```python
from build123d import *

# Parameters (mm, degrees)
SKETCH1_R                                      = 19.05
BOSS_EXTRUDE1_DEPTH                            = 9.525
SKETCH2_W                                      = 1.89865
SKETCH2_H                                      = 43.65625
F_10_CLEARANCE_HOLE1_D                         = 5.1054
F_10_CLEARANCE_HOLE1_DEPTH                     = 11.90625
F_10_CLEARANCE_HOLE2_D                         = 5.1054
F_10_CLEARANCE_HOLE2_DEPTH                     = 11.90625
F_10_24_TAPPED_HOLE2_D                         = 3.7973
F_10_24_TAPPED_HOLE3_D                         = 3.7973
F_10_24_TAPPED_HOLE3_DEPTH                     = 14.986
F_10_24_TAPPED_HOLE3_TIP                       = 1.140824014
CBORE_FOR_8_SOCKET_HEAD_CAP_SCREW1_D           = 4.9149
CBORE_FOR_8_SOCKET_HEAD_CAP_SCREW1_CBORE_D     = 7.9375
CBORE_FOR_8_SOCKET_HEAD_CAP_SCREW1_CBORE_DEPTH = 16.8656
CBORE_FOR_8_SOCKET_HEAD_CAP_SCREW2_D           = 4.9149
CBORE_FOR_8_SOCKET_HEAD_CAP_SCREW2_CBORE_D     = 7.9375
CBORE_FOR_8_SOCKET_HEAD_CAP_SCREW2_CBORE_DEPTH = 5.4356
F_8_32_TAPPED_HOLE1_D                          = 3.4544
F_8_32_TAPPED_HOLE1_DEPTH                      = 12.446
F_8_32_TAPPED_HOLE1_TIP                        = 1.037806461
F_8_32_TAPPED_HOLE2_D                          = 3.4544


with BuildPart() as part:
    # Sketch1 → Boss-Extrude1 (new body)
    with BuildSketch(Plane(origin=(0, 0, 0), x_dir=(1, 0, 0), z_dir=(0, 1, 0))):
        with BuildLine():
            Line((120.206642486, 6.011694636), (120.206642486, 17.917944636))
            Line((120.206642486, 17.917944636), (110.631837795, 17.917944636))
            ThreePointArc((110.631837795, 17.917944636), (97.981642486, 18.711694636), (110.631837795, 19.505444636))
            Line((110.631837795, 19.505444636), (120.206642486, 19.505444636))
            Line((120.206642486, 19.505444636), (120.206642486, 31.411694636))
            Line((120.206642486, 31.411694636), (-438.593357514, 31.411694636))
            Line((-438.593357514, 31.411694636), (-438.593357514, 19.505444636))
            Line((-438.593357514, 19.505444636), (-429.018552824, 19.505444636))
            ThreePointArc((-429.018552824, 19.505444636), (-416.368357514, 18.711694636), (-429.018552824, 17.917944636))
            Line((-429.018552824, 17.917944636), (-438.593357514, 17.917944636))
            Line((-438.593357514, 17.917944636), (-438.593357514, 6.011694636))
            Line((-438.593357514, 6.011694636), (37.656642486, 6.011694636))
            Line((37.656642486, 6.011694636), (37.656642486, -25.738305364))
            Line((37.656642486, -25.738305364), (94.806642486, -25.738305364))
            Line((94.806642486, -25.738305364), (94.806642486, 6.011694636))
            Line((94.806642486, 6.011694636), (120.206642486, 6.011694636))
        make_face()
        with Locations(Location((66.231642486, 2.836694636, 0), (0, 0, 90))):
            Circle(SKETCH1_R, mode=Mode.SUBTRACT)
    extrude(amount=BOSS_EXTRUDE1_DEPTH)

    # Sketch2 → #10-24 Tapped Hole1 (revolve, cut)
    with BuildSketch(Plane(origin=(115.444142486, 4.7625, -17.917944636), x_dir=(0, 1, 0), z_dir=(1, 0, 0))):
        with Locations((0.949325, 21.828125)):
            Rectangle(SKETCH2_W, SKETCH2_H)
    revolve(axis=Axis((115.444142486, 4.7625, -24.267944636), (0, 0, 1)), mode=Mode.SUBTRACT)

    # #10 Clearance Hole1
    with Locations(Plane(origin=(0, 0, -31.411694636), x_dir=(-1, 0, 0), z_dir=(0, 0, -1))):
        with Locations((-115.444142486, 4.7625)):
            Hole(F_10_CLEARANCE_HOLE1_D / 2, depth=F_10_CLEARANCE_HOLE1_DEPTH)

    # #10 Clearance Hole2
    with Locations(Plane(origin=(0, 0, -31.411694636), x_dir=(-1, 0, 0), z_dir=(0, 0, -1))):
        with Locations((433.830857514, 4.7625)):
            Hole(F_10_CLEARANCE_HOLE2_D / 2, depth=F_10_CLEARANCE_HOLE2_DEPTH)

    # #10-24 Tapped Hole2 (through all)
    with Locations(Plane(origin=(0, 0, -17.917944636), x_dir=(-1, 0, 0), z_dir=(0, 0, -1))):
        with Locations((433.830857514, 4.7625)):
            Hole(F_10_24_TAPPED_HOLE2_D / 2)

    # #10-24 Tapped Hole3
    with Locations(Plane(origin=(0, 0, 0), x_dir=(-1, 0, 0), z_dir=(0, -1, 0))):
        with Locations((-89.802842486, 26.407894636), (-42.660442486, 26.407894636), (-42.660442486, -20.734505364), (-89.802842486, -20.734505364)):
            Hole(F_10_24_TAPPED_HOLE3_D / 2, depth=F_10_24_TAPPED_HOLE3_DEPTH)
            with Locations((0, 0, -(F_10_24_TAPPED_HOLE3_DEPTH + F_10_24_TAPPED_HOLE3_TIP / 2))):  # 118° drill point
                Cone(0, F_10_24_TAPPED_HOLE3_D / 2, F_10_24_TAPPED_HOLE3_TIP, mode=Mode.SUBTRACT)

    # CBORE for #8 Socket Head Cap Screw1 (through all)
    with Locations(Plane(origin=(0, 0, -31.411694636), x_dir=(-1, 0, 0), z_dir=(0, 0, -1))):
        with Locations((-31.306642486, 4.7625), (-18.606642486, 4.7625), (406.843357514, 4.7625), (394.143357514, 4.7625)):
            CounterBoreHole(CBORE_FOR_8_SOCKET_HEAD_CAP_SCREW1_D / 2, CBORE_FOR_8_SOCKET_HEAD_CAP_SCREW1_CBORE_D / 2, CBORE_FOR_8_SOCKET_HEAD_CAP_SCREW1_CBORE_DEPTH)

    # CBORE for #8 Socket Head Cap Screw2 (through all)
    with Locations(Plane(origin=(0, 0, 0), x_dir=(-1, 0, 0), z_dir=(0, -1, 0))):
        with Locations((371.918357514, 10.774194636), (298.258357514, 10.774194636), (224.598357514, 10.774194636), (150.938357514, 10.774194636), (77.278357514, 10.774194636), (3.618357514, 10.774194636)):
            CounterBoreHole(CBORE_FOR_8_SOCKET_HEAD_CAP_SCREW2_D / 2, CBORE_FOR_8_SOCKET_HEAD_CAP_SCREW2_CBORE_D / 2, CBORE_FOR_8_SOCKET_HEAD_CAP_SCREW2_CBORE_DEPTH)

    # #8-32 Tapped Hole1
    with Locations(Plane(origin=(0, 0, 0), x_dir=(-1, 0, 0), z_dir=(0, -1, 0))):
        with Locations((371.918357514, 25.061694636), (298.258357514, 25.061694636), (224.598357514, 25.061694636), (150.938357514, 25.061694636), (77.278357514, 25.061694636), (3.618357514, 25.061694636)):
            Hole(F_8_32_TAPPED_HOLE1_D / 2, depth=F_8_32_TAPPED_HOLE1_DEPTH)
            with Locations((0, 0, -(F_8_32_TAPPED_HOLE1_DEPTH + F_8_32_TAPPED_HOLE1_TIP / 2))):  # 118° drill point
                Cone(0, F_8_32_TAPPED_HOLE1_D / 2, F_8_32_TAPPED_HOLE1_TIP, mode=Mode.SUBTRACT)

    # #8-32 Tapped Hole2 (through all)
    with Locations(Plane(origin=(0, 9.525, 0), x_dir=(1, 0, 0), z_dir=(0, 1, 0))):
        with Locations((113.856642486, 9.186694636), (94.806642486, 28.236694636), (-413.193357514, 28.236694636), (-432.243357514, 9.186694636)):
            Hole(F_8_32_TAPPED_HOLE2_D / 2)


solid = part.part
```
Part model, mm, in its own coordinate system. A direction names the side the tool comes from. Coordinates: 2 decimals unless noted, no trailing zeros. Order: outer loops, then holes, each group sorted by start corner. A loop starts at its lowest first (then second) coordinate and runs counter-clockwise, first axis right, second up. Notation, with made-up numbers: (16.25, -4) - (40.25, -4) arc R24 ccw to (40.25, 12) - close; hole circle Ø6 at (59.5, -28). An arc over 180 degrees is marked (long way). Return JSON: item names as keys, results as strings. Group by question number.
Item 1: Pull direction X, two halves, no side cores. Call faces 6 (the face through (120.207, 5, -12)), 7 (the face through (-416.374, 4.696, -18.98)), 8 (the face through (-163, 9.525, -16)): pulls with the +X half, pulls with the -X half, needs draft (parallel to the pull), parting line crosses it, or undercut.
Item 2: Drill centre lines: probe 1 along X at (y, z) = (1.75, -3); probe 2 along Z at (x, y) = (-321.5, 4); probe 3 along X at (y, z) = (7, 3). Where is each one in solid material? Low to high. Write a range as from..to.
Item 3: Cut at B-B (x = -266). List the corners of the cut face in (y, z) (3 decimals).
Item 4: Pin check, flat tips, straight feed: pin 1 (3 mm diameter, centred on x = -3.62, z = -25.06, fed in from -Y); pin 2 (2.5 mm diameter, centred on x = -300, z = -12.5, fed in from -Y); pin 3 (3 mm diameter, centred on x = -115.5, y = 2, fed in from +Z); pin 4 (3 mm diameter, centred on y = 5, z = 19.5, fed in from +X). Stop position of each tip, or through.
Item 5: Cut at A-A (z = 9). List the corners of the cut face in (x, y) (3 decimals).
Item 6: Which spindle directions (+Z, -Z, +X, -X, +Y, -Y) get a long thin tool onto all of the face, cutting with end or side? Do faces 1 (the face through (115, 7, -17.918)), 2 (the face through (37.657, 5, 10)), 3 (the face through (94.807, 5, 10)), 4 (the face through (-434, 7, -17.918)), 5 (the face through (-438.593, 5, -12)). Say none if no direction does.
Check values:
{
 "1": {"face 6": "pulls with the +X half", "face 7": "undercut", "face 8": "needs draft"},
 "2": {"probe 1": "x = 37.66..47.18, 85.28..94.81", "probe 2": "z = -31.41..-6.01", "probe 3": "x = 37.66..48.1, 84.37..94.81"},
 "3": {"outline": "(0, -31.412) - (9.525, -31.412) - (9.525, -6.012) - (0, -6.012) - close"},
 "4": {"pin 1": "passes through", "pin 2": "stops at y = 5.44", "pin 3": "stops at z = -6.01", "pin 4": "stops at x = 94.81"},
 "5": {"outline": "(37.657, 0) - (51.305, 0) - (51.305, 9.525) - (37.657, 9.525) - close; (81.158, 0) - (94.807, 0) - (94.807, 9.525) - (81.158, 9.525) - close"},
 "6": {"face 1": "+X, +Y, -Y", "face 2": "+Z, -X, +Y, -Y", "face 3": "+Z, +X, +Y, -Y", "face 4": "-X, +Y, -Y", "face 5": "+Z, -Z, -X, +Y, -Y"}
}
